Geometry: see drawing. Coordinates: mm, zero at the bounding-box minimum. Give positions to 0.01 mm unless a question says otherwise; leave off trailing zeros. Loops run counter-clockwise (first coordinate to the right, second up) from the corner with the lowest first, then second, coordinate; pieces in that order, holes last. Notation, with made-up numbers: M -1.75,78.5 L 34.25,78.5 A17 ccw 34.25,96.5 Z; hole C 61,74 d8. An arc over 180 degrees is marked long. Put each result on its own line as item: value.
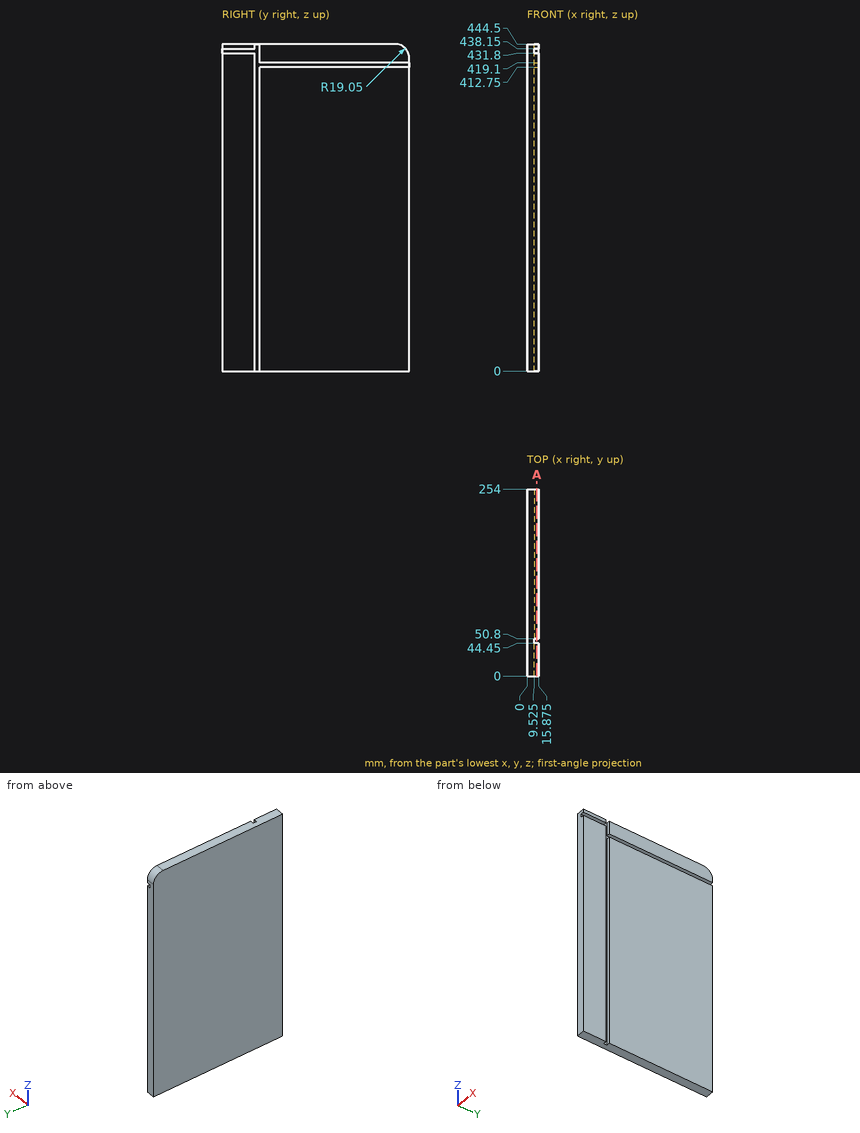
Item 1: Pin query (flat end, axial travel): pin 1 Ø1.9 at (x, z) = (11.5, 436.5) entering from -Y; pin 2 Ø3 at (x, z) = (13.5, 440) entering from +Y. Return the tip coordinate at first contact, or that it passes through.
Output values:
pin 1: y = 50.8
pin 2: y = 248.83
Item 2: Section A-A on x = 13.25. Output: boundary loops of the cut face in (y, z), then the cut area to 3 significant figures.
Output values:
outline: M 0,0 L 44.45,0 L 44.45,431.8 L 0,431.8 Z; M 0,438.15 L 44.45,438.15 L 44.45,444.5 L 0,444.5 Z; M 50.8,0 L 254,0 L 254,412.75 L 50.8,412.75 Z; M 50.8,419.1 L 254,419.1 L 254,425.45 A19.05 ccw 234.95,444.5 L 50.8,444.5 Z
area: 108,000 mm²
Item 3: Line query: probe 1 along Y at (x, z) = (11, 109); probe 2 along Z at (x, y) = (11.75, 82.5); probe 3 along Z at (x, y) = (13, 34). Output: solid intervals per line, ascending. Write a range as [from, to].
Output values:
probe 1: [0, 44.45], [50.8, 254]
probe 2: [0, 412.75], [419.1, 444.5]
probe 3: [0, 431.8], [438.15, 444.5]
